Autodesk Inventor part; units mm, degrees
ref_plane "YZ Plane" through (0, 0, 0) normal (1, 0, 0) x (0, 1, 0)
ref_plane "XZ Plane" through (0, 0, 0) normal (0, 1, 0) x (-1, 0, 0)
ref_plane "XY Plane" through (0, 0, 0) normal (0, 0, 1) x (1, 0, 0)
sketch "Sketch1" plane through (0, 0, 0) normal (0, 1, 0) x (-1, 0, 0)
  line L0 (60, -60) -> (-60, -60)
  line L1 (-60, -60) -> (-60, 60)
  line L2 (-60, 60) -> (60, 60)
  line L3 (60, 60) -> (60, -60)
  point P0 (0, 0)
  dimension "d0" = 120
  dimension "d1" = 120
  dimension "d2" = 60
  dimension "d3" = 60
extrude "Extrusion1" add sketch "Sketch1" along normal blind 5
sketch "Sketch2" plane through (0, 5, 0) normal (0, 1, 0) x (1, 0, 0)
  line L0 (-40, 40) -> (-60, 40)
  line L1 (-60, 40) -> (-60, 60)
  line L2 (-60, 60) -> (-40, 60)
  line L3 (-40, 60) -> (-40, 40)
  line L4 (60, -60) -> (40, -60)
  line L5 (40, -60) -> (40, -40)
  line L6 (40, -40) -> (60, -40)
  line L7 (60, -40) -> (60, -60)
  line L8 (60, 60) -> (60, -60)
  line L9 (-60, -60) -> (60, -60)
  line L10 (60, 60) -> (-60, 60)
  line L11 (60, 60) -> (40, 60)
  line L12 (40, 60) -> (40, 40)
  line L13 (40, 40) -> (60, 40)
  line L14 (60, 40) -> (60, 60)
  line L15 (-60, 60) -> (-60, -60)
  line L16 (-60, -60) -> (-40, -60)
  line L17 (-40, -60) -> (-40, -40)
  line L18 (-40, -40) -> (-60, -40)
  line L19 (-60, -40) -> (-60, -60)
  point P0 (0, 0)
  dimension "d6" = 20
  dimension "d7" = 20
  dimension "d8" = 20
  dimension "d9" = 20
  dimension "d10" = 0
  dimension "d11" = 0
  dimension "d12" = 20
  dimension "d13" = 20
  dimension "d14" = 20
  dimension "d15" = 20
extrude "Extrusion2" add sketch "Sketch2" along normal blind 40 contours L0 L1 L2 L3 | L18 L17 L9 L15 | L10 L8 L13 L12 | L5 L6 L7 L4
equation "\"d1\" = d0"
equation "\"d7\" = d6"
equation "\"d8\" = d6"
equation "\"d9\" = d6"
equation "\"d12\" = d6"
equation "\"d13\" = d6"
equation "\"d14\" = d6"
equation "\"d15\" = d6"
properties part number "FalseFloor" material "ABS Plastic"
Here's how the part is built. I have some questions about the finished solid (model axes, mm). A direction names the side the tool comes from. Coordinates: 2 decimals unless noted, no trailing zeros. Order: outer loops, then holes, each group sorted by start corner. A loop starts at its lowest first (then second) coordinate and runs counter-clockwise, first axis right, second up. Notation, with made-up numbers: (38, -21.75) -> (51, -21.75) arc R25 ccw to (51, 17.25) -> close; hole circle Ø5 at (34.5, 10.5). An arc over 180 degrees is marked (long way). Return JSON: item names as keys, results as strings.
1) If we section it at B-B on z = 48.5: List the corners of the cut face in (x, y) for me.
Conclusion:
{"outline": "(-60, 0) -> (60, 0) -> (60, 45) -> (40, 45) -> (40, 5) -> (-40, 5) -> (-40, 45) -> (-60, 45) -> close"}
2) If we section it at D-D on x = -3: List the corners of the cut face in (y, z) for me.
Conclusion:
{"outline": "(0, -60) -> (5, -60) -> (5, 60) -> (0, 60) -> close"}
3) If we section it at A-A on y = 24.5: List the corners of the cut face in (x, z) for me, plus the area to 3 significant figures.
Conclusion:
{"outline": "(-60, -60) -> (-40, -60) -> (-40, -40) -> (-60, -40) -> close; (-60, 40) -> (-40, 40) -> (-40, 60) -> (-60, 60) -> close; (40, -60) -> (60, -60) -> (60, -40) -> (40, -40) -> close; (40, 40) -> (60, 40) -> (60, 60) -> (40, 60) -> close", "area": "1,600 mm²"}
4) Thinking about a two-plate mould opening in X: for faces 1 (the flat face through (1, 5, 1)), 2 (the flat face through (60, 2, -14)), 3 (the flat face through (50, 45, 50)), which applies, +X half, -X half, draft (parallel to the pull), parting line (faces both ways), or undercut?
Conclusion:
{"face 1": "undercut", "face 2": "+X half", "face 3": "draft"}
5) If we section it at C-C on x = 42.5: List the corners of the cut face in (y, z) for me.
Conclusion:
{"outline": "(0, -60) -> (45, -60) -> (45, -40) -> (5, -40) -> (5, 40) -> (45, 40) -> (45, 60) -> (0, 60) -> close"}
6) On a 3-axis mill with a long thin cutter (end or side, diameter ignored), from which of +Z, -Z, +X, -X, +Y, -Y can I reach the whole of each face in a straight line? I mean faces 4 (the flat face through (50, 45, -50)), 5 (the flat face through (50, 25, 40)), 6 (the flat face through (-40, 25, 50)). Say none if no direction works.
Conclusion:
{"face 4": "+Z, -Z, +X, -X, +Y", "face 5": "+X, -X, +Y", "face 6": "+Z, -Z, +Y"}
7) If I drill on probe 1 along X at (y, z) = (38.5, 53.5); probe 2 along Y at (x, z) = (52, -30), over which ranges is the centre line in solid material (lowest first)?
Conclusion:
{"probe 1": "x = -60 to -40, 40 to 60", "probe 2": "y = 0 to 5"}
8) I'm going to push a flat-ended pin straight in: P1, Ø2, axis at x = -26.5, z = 18, coming from the +Y side. Where does the tip first touch, or does it pass through?
Conclusion:
{"P1": "stops at y = 5"}
